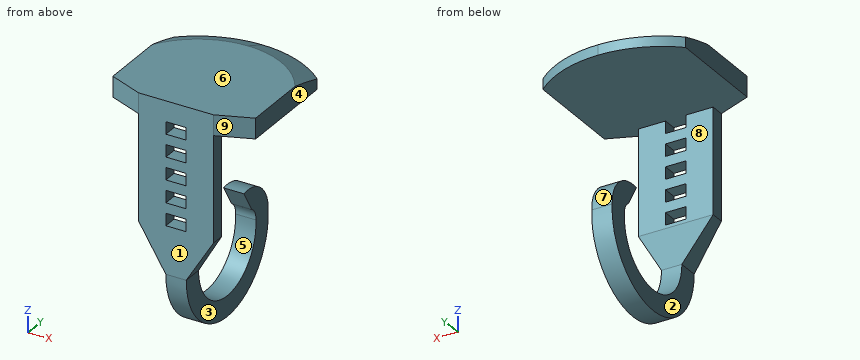
from build123d import *

# Parameters (mm, degrees)
F1_DEPTH    = 6
F2_W        = 8
F2_H        = 4
F3_DEPTH    = 36
F4_DEPTH    = 4
F5_C1_SIZE2 = 10
F5_C1_SIZE  = 4
F5_C2_SIZE2 = 10
F5_C2_SIZE  = 4
F6_W        = 4
F6_H        = 3
F7_DEPTH    = 6
F10_DEPTH   = 3
F11_W       = 14
F11_H       = 4
F11_W_2     = 8
F12_DEPTH   = 1
F12_FACE_W  = 22
F12_FACE_H  = 4
F10_FACE_W  = 6
F10_FACE_H  = 6
F15_DEPTH   = 109
F16_SIZE2   = 3
F16_SIZE    = 7


# Not quite as in the source:
# - an extrude ends at something that could not be found from the text; its depth is read off the source's solid


with BuildPart() as f1:
    # F0 (on Top) → F1 (new body)
    with BuildSketch(Plane.XY):
        with BuildLine():
            ThreePointArc((4.2292630374, 28.5867799968), (-5.5346345873, 34.5190491883), (-16.7707372875, 36.5867799968))
            ThreePointArc((-16.7707372875, 36.5867799968), (-28.0068396415, 34.5190490726), (-37.7707369626, 28.5867799968))
            Line((-37.7707369626, 28.5867799968), (-37.7707369626, -1.4132200032))
            Line((-37.7707369626, -1.4132200032), (4.2292630374, -1.4132200032))
            Line((4.2292630374, -1.4132200032), (4.2292630374, 28.5867799968))
        make_face()
    extrude(amount=F1_DEPTH)

    # F2 (on face) → F3 (join)
    with BuildSketch(Plane.XY.offset(6)):
        with Locations((-23.7707369626, -3.4132200032)):
            Rectangle(F2_W, F2_H)
        with Locations((-9.7707369626, -3.4132200032)):
            Rectangle(F2_W, F2_H)
    extrude(amount=-F3_DEPTH)

    # F4 (add): faces of the model
    f4_faces = [f1.faces().sort_by_distance(p)[0] for p in [
        (-32.7707369626, -1.4132200032, 3),
        (-0.7707369626, -1.4132200032, 3),
        (-16.7707369626, -1.4132200032, 3),
    ]]
    extrude(f4_faces, amount=F4_DEPTH)

    # F5: chamfer of 10 x 4 on 2 edges, made by hand

    # F5_c1
    f5_c1_edges = [f1.edges().sort_by_distance(p)[0] for p in [
        (-37.7707369626, -5.4132200032, 3),
    ]]
    f5_c1_side = f1.faces().sort_by_distance((-37.7707369626, -5.3332200032, 3))[0]
    chamfer(f5_c1_edges, length=F5_C1_SIZE, length2=F5_C1_SIZE2, reference=f5_c1_side)

    # F5_c2
    f5_c2_edges = [f1.edges().sort_by_distance(p)[0] for p in [
        (4.2292630374, -5.4132200032, 3),
    ]]
    f5_c2_side = f1.faces().sort_by_distance((4.2292630374, -5.3332200032, 3))[0]
    chamfer(f5_c2_edges, length=F5_C2_SIZE, length2=F5_C2_SIZE2, reference=f5_c2_side)

    # F6 (on face) → F7 (join, through all)
    with BuildSketch(Plane(origin=(-13.7707369626, 0, 0), x_dir=(0, -1, 0), z_dir=(-1, 0, 0))):
        with Locations((3.4132200032, -24.9)):
            Rectangle(F6_W, F6_H)
        with Locations((3.4132200032, -18.3)):
            Rectangle(F6_W, F6_H)
        with Locations((3.4132200032, -11.7)):
            Rectangle(F6_W, F6_H)
        with Locations((3.4132200032, -5.1)):
            Rectangle(F6_W, F6_H)
    extrude(amount=F7_DEPTH)

    # F11 (on face) → F12 (join)
    with BuildSketch(Plane(origin=(0, 0, -30), x_dir=(1, 0, 0), z_dir=(0, 0, -1))):
        with Locations((-12.7707369626, 3.4132200032)):
            Rectangle(F11_W, F11_H)
        with Locations((-23.7707369626, 3.4132200032)):
            Rectangle(F11_W_2, F11_H)
    extrude(amount=F12_DEPTH)



with BuildPart() as f10:
    # F9 (on line) → F10 (new body, symmetric)
    with BuildSketch(Plane.YZ.offset(-16.7707369626)):
        with BuildLine():
            ThreePointArc((-5.4132200032, -44), (15.1917157006, -63.9908492264), (34.5501852762, -42.7906821553))
            ThreePointArc((34.5501852762, -42.7906821553), (24.5246696764, -32.3338991708), (14.5746107682, -42.8625078704))
            Line((14.5746107682, -42.8625078704), (20.5957170737, -42.8625078704))
            ThreePointArc((20.5957170737, -42.8625078704), (24.5244376896, -38.3339982315), (28.5344518581, -42.7906821553))
            ThreePointArc((28.5344518581, -42.7906821553), (15.1920047243, -57.9869118475), (0.5867799968, -44))
            Line((0.5867799968, -44), (-5.4132200032, -44))
        make_face()
    extrude(amount=F10_DEPTH, both=True)


with BuildPart() as f1_1:
    add(f1.part)

    add(f10.part)  # F13 merges F10
    # F12_face (on face) → F13 section 0
    with BuildSketch(Plane(origin=(-16.7707369626, -3.4132200032, -31), x_dir=(1, 0, 0), z_dir=(0, 0, -1))):
        Rectangle(F12_FACE_W, F12_FACE_H)
    # F10_face (on face) → F13 section 1
    with BuildSketch(Plane(origin=(-16.7707369626, -2.4132200032, -44), x_dir=(1, 0, 0), z_dir=(0, 0, 1))):
        Rectangle(F10_FACE_W, F10_FACE_H)
    loft()

    # F14 (on face) → F15 (cut, through all)
    with BuildSketch(Plane.YZ.offset(-13.7707369626)):
        with BuildLine():
            Line((22.7304068946, -32.502746223), (21.8552816659, -31.0546644032))
            Line((21.8552816659, -31.0546644032), (14.088241172, -33.6755602773))
            Line((14.088241172, -33.6755602773), (14.5746107682, -42.8625078704))
            ThreePointArc((14.5746107682, -42.8625078704), (16.7033355644, -36.1481265127), (22.7304068946, -32.502746223))
        make_face()
        with BuildLine():
            Line((26.5877404927, -38.885529479), (22.7304068946, -32.502746223))
            ThreePointArc((22.7304068946, -32.502746223), (16.7033355644, -36.1481265127), (14.5746107682, -42.8625078704))
            Line((14.5746107682, -42.8625078704), (20.5957170737, -42.8625078704))
            ThreePointArc((20.5957170737, -42.8625078704), (22.3486471202, -39.0010956404), (26.5877404927, -38.885529479))
        make_face()
    extrude(amount=-F15_DEPTH, mode=Mode.SUBTRACT)

    # F16
    f16_edges = [f1_1.edges().sort_by_distance(p)[0] for p in [
        (-16.770737, 36.58678, 6),
    ]]
    f16_side = f1_1.faces().sort_by_distance((-16.770737, 14.854781, 6))[0]
    chamfer(f16_edges, length=F16_SIZE, length2=F16_SIZE2, reference=f16_side)


solid = f1_1.part
Verification items for the finished model (mm, model axes). Face numbers are marked on the shaded views. A direction names the side the tool comes from. Give positions to 0.01 mm unless a question says otherwise; leave off trailing zeros. Loops run counter-clockwise (first coordinate to the right, second up) from the corner with the lowest first, then second, coordinate; pieces in that order, holes last.
1) Draft check along Z on the marked faces 6, 7, 8 and 9. Enter one of: pulls with the +Z half, pulls with the -Z half, needs draft (parallel to the pull), parting line crosses it, or undercut.
2) Sectioned sample at C-C, the plane x = -15. Count the separate pieces of the cut face and the enclosed holes in it, then the cut area to 3 significant figures.
3) Sectioned sample at B-B, the plane y = 8. Enter the section's corners in (x, z), then the cut area to 3 significant figures.
4) Depth check by flat-ended pin: pin 1 Ø1.8 at (y, z) = (-3, -14.5) entering from +X; pin 2 Ø2 at (y, z) = (-3.5, -13) entering from -X; pin 3 Ø4.5 at (x, y) = (-18, -3.5) entering from -Z; pin 4 Ø6 at (x, z) = (-10, -56.5) entering from +Y. Enter the tip coordinate at first touch or a pass-through.
5) Sectioned sample at A-A, the plane z = -22. Enter the section's corners in (x, y), then the cut area to 3 significant figures.
6) Set-up check for the marked faces 1, 2, 3, 4 and 5: record each of +Z, -Z, +X, -X, +Y, -Y from which the full face is reachable in a straight line by a thin tool's end or side.
7) Thickness scan on line 1 along Z through (x, y) = (-20.5, 19); line 2 along X through (y, z) = (2, -54); line 3 along Y through (x, z) = (-23, -19). Record the ranges inside material, lowest first.
Answers:
1. face 6: pulls with the +Z half
1. face 7: undercut
1. face 8: undercut
1. face 9: needs draft
2. separate pieces: 6
2. enclosed holes: 0
2. area: 755 mm2
3. outline: (-37.77, 0) - (4.23, 0) - (4.23, 6) - (-37.77, 6) - close; (-19.77, -62.88) - (-13.77, -62.88) - (-13.77, -56.35) - (-19.77, -56.35) - close
3. area: 291 mm2
4. pin 1: stops at x = -5.77
4. pin 2: stops at x = -27.77
4. pin 3: stops at z = -56.21
4. pin 4: passes through
5. outline: (-27.77, -5.41) - (-19.77, -5.41) - (-19.77, -1.41) - (-27.77, -1.41) - close; (-13.77, -5.41) - (-5.77, -5.41) - (-5.77, -1.41) - (-13.77, -1.41) - close
5. area: 64.0 mm2
6. face 1: +Z, -Z, +X, -X, -Y
6. face 2: -Z, -X, +Y
6. face 3: -Z, +X, +Y
6. face 4: +Z, -Z, +X, +Y, -Y
6. face 5: +X, -X
7. line 1: z = 0 to 6
7. line 2: x = -19.77 to -13.77
7. line 3: y = -5.41 to -1.41
